Build history of the part. All positions in model axes, mm. Face numbers are marked on the shaded views. Round coordinates to 2 decimals unless told otherwise and drop trailing zeros. Write each loop counter-clockwise with the first axis right and the second up, starting at its lowest first coordinate (ties: lowest second). Pieces come first, ordered by that corner, then holes. Notation, with made-up numbers: M 38,6 L 79,6 A32 cw 79,32 Z; hole C 48,16.25 d7. An arc over 180 degrees is marked long. Use a Markdown table: item, result.
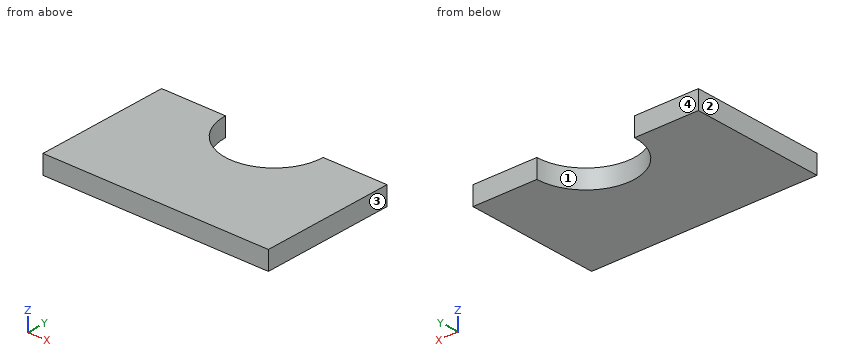
from build123d import *

# Parameters (mm, degrees)
F1_DEPTH = 6.35


with BuildPart() as f1:
    # F0 (on Top) → F1 (new body)
    with BuildSketch(Plane.XY):
        with BuildLine():
            Line((21.59, 0), (0, 0))
            Line((0, 0), (0, -45.4025))
            Line((0, -45.4025), (76.2, -45.4025))
            Line((76.2, -45.4025), (76.2, 0))
            Line((76.2, 0), (54.61, 0))
            ThreePointArc((54.61, 0), (38.1, -16.51), (21.59, 0))
        make_face()
    extrude(amount=F1_DEPTH)


solid = f1.part
Q1. Drill centre lines: L1, parallel to X at y = -7, z = 4.5; L2, parallel to Y at x = 38, z = 5; L3, parallel to X at y = -3.5, z = 4.5. Where is each one in solid material? Low to high.
Response values:
| item | result |
|---|---|
| L1 | x = 0 to 23.15, 53.05 to 76.2 |
| L2 | y = -45.4 to -16.51 |
| L3 | x = 0 to 21.97, 54.23 to 76.2 |
Q2. Cut at C-C on x = 48. Give the cut face in (y, z), and give its area (3 significant figures).
Response values:
| item | result |
|---|---|
| outline | M -45.4,0 L -13.21,0 L -13.21,6.35 L -45.4,6.35 Z |
| area | 204 mm2 |
Q3. Cut at A-A on z = 4.25. Give the cut face in (x, y), and give its area (3 significant figures).
Response values:
| item | result |
|---|---|
| outline | M 0,-45.4 L 76.2,-45.4 L 76.2,0 L 54.61,0 A16.51 cw 21.59,0 L 0,0 Z |
| area | 3,030 mm2 |
Q4. Two-plate mould, pull along X, no slides. Class the marked faces 1, 2, 3 and 4: +X half, -X half, draft (parallel to the pull), parting line (faces both ways), or undercut.
Response values:
| item | result |
|---|---|
| face 1 | undercut |
| face 2 | -X half |
| face 3 | +X half |
| face 4 | draft |
Q5. Cut at B-B on x = 38.1. Give the cut face in (y, z).
Response values:
| item | result |
|---|---|
| outline | M -45.4,0 L -16.51,0 L -16.51,6.35 L -45.4,6.35 Z |
